Check sheet for the drawn part. Datum: minimum x, y, z corner. Units: mm. Give positions to 0.01 mm unless a question says otherwise; leave off trailing zeros. Write each loop counter-clockwise with the first axis right and the second up, starting at its lowest first coordinate (ties: lowest second). Pieces come first, ordered by that corner, then holes. Notation, with made-up numbers: (42, 32) -> (85, 32) arc R12 ccw to (85, 49) -> close; hole circle Ø1 at (-3, -13.5). An arc over 180 degrees is marked (long way). Write item = value, one per line. Start each with the question number.
1. Depth check by flat-ended pin: P1, Ø1.5, axis at x = 84, z = 3.5, coming from the -Y side; P2, Ø3, axis at y = 110.5, z = 3, coming from the -X side; P3, Ø5, axis at x = 135.5, z = 3.5, coming from the +Y side; P4, Ø1, axis at y = 179.5, z = 5.5, coming from the -X side. Enter the tip coordinate at first touch or a pass-through.
2. Cross-section at A-A, the plane z = 7.5. Record the cut outline in (x, y), plus the area to 3 significant figures.
3. Cross-section at B-B, the plane x = 97. Record the cut outline in (y, z).
4. Cross-section at C-C, the plane y = 53. Record the cut outline in (x, z), plus the area to 3 significant figures.
5. Thickness scan on line 1 along Y through (x, z) = (134, 0.75); line 2 along X through (y, z) = (193, 7.75) (1 decimal); line 3 along Y through (x, z) = (32, 4.25) (1 decimal). Record the ranges inside material, lowest first.
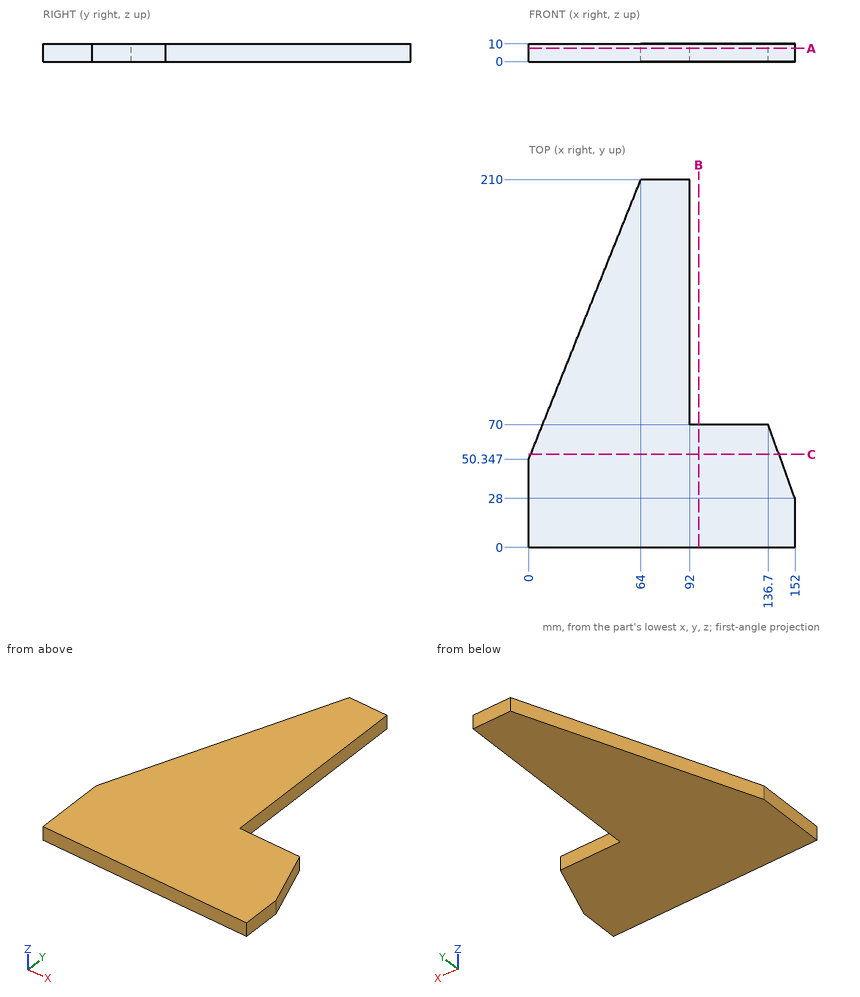
Answers:
q1.P1 = 0
q1.P2 = 23.51
q1.P3 = 70
q1.P4 = 51.57
q2.outline = (0, 0) -> (152, 0) -> (152, 28) -> (136.7, 70) -> (92, 70) -> (92, 210) -> (64, 210) -> (0, 50.35) -> close
q2.area = 18,100 mm^2
q3.outline = (0, 0) -> (70, 0) -> (70, 10) -> (0, 10) -> close
q4.outline = (1.06, 0) -> (142.89, 0) -> (142.89, 10) -> (1.06, 10) -> close
q4.area = 1,420 mm^2
q5.line_1 = 0 to 70
q5.line_2 = 57.2 to 92
q5.line_3 = 0 to 130.2
